Source: CAD feature listing. Evaluate the final solid. Frame: model axes, mm. Coordinates: 2 decimals unless noted, no trailing zeros. Order: outer loops, then holes, each group sorted by start corner. A loop starts at its lowest first (then second) coordinate and runs counter-clockwise, first axis right, second up.
```python
from build123d import *

# Parameters (mm, degrees)
SKETCH_1_W          = 6.35
SKETCH_1_H          = 7.9375
HOLE_WIZARD_1_D     = 6.35
HOLE_WIZARD_1_DEPTH = 7.9375
SKETCH_4_W          = 2.413
SKETCH_4_H          = 4.286494245
FILLET_1_R          = 0.127


with BuildPart() as part:
    # 草图1 → 旋转1 (revolve)
    with BuildSketch(Plane(origin=(0, 0, 0), x_dir=(-1, 0, 0), z_dir=(0, 0, -1))):
        with Locations((-3.175, 0)):
            Rectangle(SKETCH_1_W, SKETCH_1_H)
    revolve(axis=Axis((0, -3.96875, 0), (0, 1, 0)))

    # 孔1
    with Locations(Plane(origin=(0, -3.96875, 0), x_dir=(-1, 0, 0), z_dir=(0, -1, 0))):
        with Locations((0, 0)):
            Hole(HOLE_WIZARD_1_D / 2, depth=HOLE_WIZARD_1_DEPTH)

    # 草图4 → 孔2 (revolve, cut)
    with BuildSketch(Plane(origin=(0, 0, 2.063505755), x_dir=(0, 1, 0), z_dir=(1, 0, 0))):
        with Locations((1.2065, 2.143247123)):
            Rectangle(SKETCH_4_W, SKETCH_4_H)
    revolve(axis=Axis((0, 0, 112.063505755), (0, 0, -1)), mode=Mode.SUBTRACT)

    # 圆角1
    fillet_1_edges = [part.edges().sort_by_distance(p)[0] for p in [
        (-3.175, -3.96875, 0),
        (-3.175, 3.96875, 0),
        (-6.35, 3.96875, 0),
        (-6.35, -3.96875, 0),
    ]]
    fillet(fillet_1_edges, radius=FILLET_1_R)


solid = part.part
```
1. Ray query, line 1 (X direction, y = 2.25, z = 0) (3 decimals); line 2 (Y direction, x = 0, z = 3.8); line 3 (X direction, y = 0, z = 5.4). Return the intervals inside material, ascending.
Findings:
line 1: x = -6.35 to -3.175, 3.175 to 6.35
line 2: y = -3.97 to -2.41, 2.41 to 3.97
line 3: x = -3.34 to -2.41, 2.41 to 3.34
2. Draft query along X for faces 1 (the face through (0.11, -2.41, 4.24)), 2 (the face through (3, -3.969, 3)), 3 (the face through (-0.8, 0.1, -6.3)), 4 (the face through (-0.41, 0.05, -3.15)). Return one class per face: released by +X, released by -X, zero draft, split by the parting line, or undercut.
Findings:
face 1: undercut
face 2: zero draft
face 3: split by the parting line
face 4: undercut
3. Section query D-D on y = -0.5. Return loops of the section in (x, z) (3 decimals).
Findings:
outline: (-2.361, 2.123) - (-2.361, 5.895) arc R6.35 ccw (long way) to (2.361, 5.895) - (2.361, 2.123) arc R3.175 cw (long way) to start
4. Section query B-B on x = 0. Return loops of the section in (y, z) (3 decimals), plus the area to 3 significant figures.
Findings:
outline: (-3.969, -6.223) arc R0.127 ccw to (-3.842, -6.35) - (3.842, -6.35) arc R0.127 ccw to (3.969, -6.223) - (3.969, -3.302) arc R0.127 ccw to (3.842, -3.175) - (-3.842, -3.175) arc R0.127 ccw to (-3.969, -3.302) - close; (-3.969, 3.302) arc R0.127 ccw to (-3.842, 3.175) - (-2.413, 3.175) - (-2.413, 6.35) - (-3.842, 6.35) arc R0.127 ccw to (-3.969, 6.223) - close; (2.413, 3.175) - (3.842, 3.175) arc R0.127 ccw to (3.969, 3.302) - (3.969, 6.223) arc R0.127 ccw to (3.842, 6.35) - (2.413, 6.35) - close
area: 35.1 mm2
5. Pin query (flat end, axial travel): P1, Ø4.5, axis at x = 0, y = 0, coming from the +Z side; P2, Ø1.5, axis at x = 2.5, y = 1, coming from the +Z side; P3, Ø2, axis at y = -0.5, z = -2, coming from the -X side; P4, Ø1.5, axis at y = 2, z = -0.5, coming from the +X side. Return the tip coordinate at first contact, or that it passes through.
Findings:
P1: stops at z = -2.24
P2: stops at z = 6.05
P3: stops at x = -6.27
P4: stops at x = 6.35
6. Section query A-A on z = 0. Return loops of the section in (x, y) (3 decimals).
Findings:
outline: (-6.35, -3.842) arc R0.127 ccw to (-6.223, -3.969) - (-3.302, -3.969) arc R0.127 ccw to (-3.175, -3.842) - (-3.175, 3.842) arc R0.127 ccw to (-3.302, 3.969) - (-6.223, 3.969) arc R0.127 ccw to (-6.35, 3.842) - close; (3.175, -3.842) arc R0.127 ccw to (3.302, -3.969) - (6.223, -3.969) arc R0.127 ccw to (6.35, -3.842) - (6.35, 3.842) arc R0.127 ccw to (6.223, 3.969) - (3.302, 3.969) arc R0.127 ccw to (3.175, 3.842) - close
7. Section query C-C on y = 3. Return loops of the section in (x, z) (3 decimals).
Findings:
outline: circle Ø12.7 at (0, 0); hole circle Ø6.35 at (0, 0)
